from build123d import *

# Parameters (mm, degrees)
F1_DEPTH  = 9.652
F2_DEPTH  = 9.652
F4_DEPTH  = 44.704
F5_R      = 10.922
F7_DEPTH  = 3.175
F9_DEPTH  = 100.5007969078
F12_DEPTH = 3.175


with BuildPart() as f1:
    # F0 (on Top) → F1 (new body)
    with BuildSketch(Plane.XY):
        with BuildLine():
            Line((83.4274074162, 44.704), (19.9274074162, 44.704))
            Line((19.9274074162, 44.704), (19.9274074162, 0))
            Line((19.9274074162, 0), (83.4274074162, 0))
            Line((83.4274074162, 0), (83.4274074162, 12.7))
            Line((83.4274074162, 12.7), (58.0274074162, 12.7))
            ThreePointArc((58.0274074162, 12.7), (48.3754074162, 22.352), (58.0274074162, 32.004))
            Line((58.0274074162, 32.004), (83.4274074162, 32.004))
            Line((83.4274074162, 32.004), (83.4274074162, 44.704))
        make_face()
    extrude(amount=F1_DEPTH)

    # F0 (on Top) → F2 (join)
    with BuildSketch(Plane.XY):
        with BuildLine():
            ThreePointArc((83.4274074162, 0), (105.7794074162, 22.352), (83.4274074162, 44.704))
            Line((83.4274074162, 44.704), (83.4274074162, 32.004))
            ThreePointArc((83.4274074162, 32.004), (93.0794074162, 22.352), (83.4274074162, 12.7))
            Line((83.4274074162, 12.7), (83.4274074162, 0))
        make_face()
    extrude(amount=F2_DEPTH)

    # F3 (on face) → F4 (join)
    with BuildSketch(Plane.XZ):
        Polygon((19.9274074162, 0), (19.9274074162, 9.652), (0.8774074162, 42.6475678842), (-7.4814697811, 37.8215678842), (14.354822618, 0), align=None)
    extrude(amount=-F4_DEPTH)

    # F5
    f5_edges = [f1.edges().sort_by_distance(p)[0] for p in [
        (-3.302031, 0, 40.234568),
        (-3.302031, 44.704, 40.234568),
    ]]
    fillet(f5_edges, radius=F5_R)

    # F6 (on face) → F7 (cut)
    with BuildSketch(Plane(origin=(19.1249941608, 0, 11.041820527), x_dir=(0, 1, 0), z_dir=(0.8660254038, 0, 0.5))):
        with BuildLine():
            Line((17.272, 25.5731734892), (10.922, 25.5731734892))
            Line((10.922, 25.5731734892), (4.572, 25.5731734892))
            ThreePointArc((4.572, 25.5731734892), (10.922, 19.2231734892), (17.272, 25.5731734892))
        make_face()
        with BuildLine():
            Line((10.922, 31.9231734892), (10.922, 25.5731734892))
            Line((10.922, 25.5731734892), (17.272, 25.5731734892))
            ThreePointArc((17.272, 25.5731734892), (15.4121280605, 30.0633015498), (10.922, 31.9231734892))
        make_face()
        with BuildLine():
            Line((4.572, 25.5731734892), (10.922, 25.5731734892))
            Line((10.922, 25.5731734892), (10.922, 31.9231734892))
            ThreePointArc((10.922, 31.9231734892), (6.4318719395, 30.0633015498), (4.572, 25.5731734892))
        make_face()
        with BuildLine():
            ThreePointArc((33.782, 31.9231734892), (29.2918719395, 30.0633015498), (27.432, 25.5731734892))
            Line((27.432, 25.5731734892), (33.782, 25.5731734892))
            Line((33.782, 25.5731734892), (33.782, 31.9231734892))
        make_face()
        with BuildLine():
            Line((33.782, 31.9231734892), (33.782, 25.5731734892))
            Line((33.782, 25.5731734892), (40.132, 25.5731734892))
            ThreePointArc((40.132, 25.5731734892), (38.2721280605, 30.0633015498), (33.782, 31.9231734892))
        make_face()
        with BuildLine():
            Line((33.782, 25.5731734892), (27.432, 25.5731734892))
            ThreePointArc((27.432, 25.5731734892), (33.782, 19.2231734892), (40.132, 25.5731734892))
            Line((40.132, 25.5731734892), (33.782, 25.5731734892))
        make_face()
    extrude(amount=-F7_DEPTH, mode=Mode.SUBTRACT)

    # F8 (on face) → F9 (cut, through all)
    with BuildSketch(Plane(origin=(10.7661169635, 0, 6.215820527), x_dir=(0, -1, 0), z_dir=(-0.8660254038, 0, -0.5))):
        with BuildLine():
            Line((-30.607, 25.5731734892), (-33.782, 25.5731734892))
            Line((-33.782, 25.5731734892), (-36.957, 25.5731734892))
            ThreePointArc((-36.957, 25.5731734892), (-33.782, 22.3981734892), (-30.607, 25.5731734892))
        make_face()
        with BuildLine():
            Line((-33.782, 25.5731734892), (-33.782, 28.7481734892))
            ThreePointArc((-33.782, 28.7481734892), (-36.0270640303, 27.8182375195), (-36.957, 25.5731734892))
            Line((-36.957, 25.5731734892), (-33.782, 25.5731734892))
        make_face()
        with BuildLine():
            ThreePointArc((-30.607, 25.5731734892), (-31.5369359697, 27.8182375195), (-33.782, 28.7481734892))
            Line((-33.782, 28.7481734892), (-33.782, 25.5731734892))
            Line((-33.782, 25.5731734892), (-30.607, 25.5731734892))
        make_face()
        with BuildLine():
            Line((-10.922, 25.5731734892), (-10.922, 28.7481734892))
            ThreePointArc((-10.922, 28.7481734892), (-13.1670640303, 27.8182375195), (-14.097, 25.5731734892))
            Line((-14.097, 25.5731734892), (-10.922, 25.5731734892))
        make_face()
        with BuildLine():
            ThreePointArc((-7.747, 25.5731734892), (-8.6769359697, 27.8182375195), (-10.922, 28.7481734892))
            Line((-10.922, 28.7481734892), (-10.922, 25.5731734892))
            Line((-10.922, 25.5731734892), (-7.747, 25.5731734892))
        make_face()
        with BuildLine():
            Line((-10.922, 25.5731734892), (-14.097, 25.5731734892))
            ThreePointArc((-14.097, 25.5731734892), (-10.922, 22.3981734892), (-7.747, 25.5731734892))
            Line((-7.747, 25.5731734892), (-10.922, 25.5731734892))
        make_face()
    extrude(amount=-F9_DEPTH, mode=Mode.SUBTRACT)

    # F11 (on offset) → F12 (join, symmetric)
    with BuildSketch(Plane.XZ.offset(-22.352)):
        Polygon((0.8774074162, 42.6475678842), (19.9274074162, 9.652), (45.3274074162, 9.652), align=None)
    extrude(amount=F12_DEPTH, both=True)


solid = f1.part
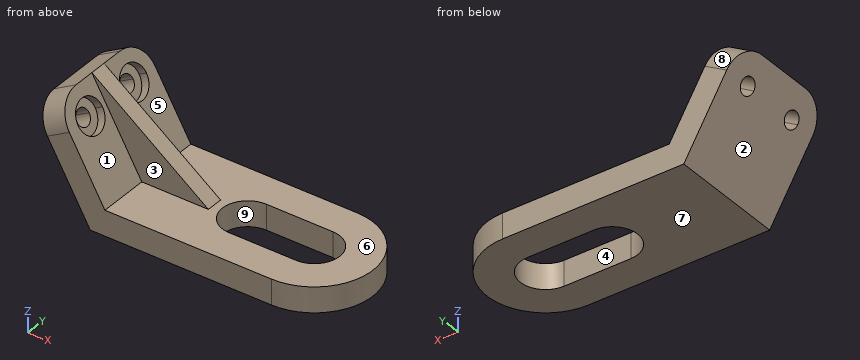
Here's how the part is built. I have some questions about the finished solid (model axes, mm). Face numbers are marked on the shaded views. A direction names the side the tool comes from. Give positions to 0.01 mm unless a question says otherwise; leave off trailing zeros. Loops run counter-clockwise (first coordinate to the right, second up) from the corner with the lowest first, then second, coordinate; pieces in that order, holes last. Notation, with made-up numbers: (11, 83.5) -> (37, 83.5) arc R20 cw to (37, 107.5) -> close; hole circle Ø9 at (-37.75, 73). An arc over 180 degrees is marked (long way). Answer as a JSON object with one key per item and string values. Group by question number.
Item 1: Thinking about a two-plate mould opening in X: for the marked faces 1, 2, 3 and 4, which applies, pulls with the +X half, pulls with the -X half, needs draft (parallel to the pull), parting line crosses it, or undercut?
Item 2: Imagine slicing it at A-A on x = 78.5. Write out the boundary of the cut face in (y, z), then the cut area to 3 significant figures.
Item 3: Imagine slicing it at B-B on y = 21. Write out the boundary of the cut face in (x, z), then the cut area to 3 significant figures.
Item 4: Imagine slicing it at D-D on x = 39.5. Write out the boundary of the cut face in (y, z).
Item 5: I need wall thicknesses on L1, parallel to Z at x = 31.5, y = 21.5; L2, parallel to Z at x = 21, y = 41; L3, parallel to Y at x = 74.5, z = 9. Which ranges of each line are inside material? Lowest first, please.
Item 6: On a 3-axis mill with a long thin cutter (end or side, diameter ignored), from which of +Z, -Z, +X, -X, +Y, -Y can I reach the whole of each face in a straight line? I mean the marked faces 5, 6, 7, 8 and 9. Say none if no direction works.
Item 7: Will these pins go through, and if not, where does the flat tip stop? pin 1 (10 mm diameter, centred on x = 30.5, z = 24.5, fed in from -Y); pin 2 (4 mm diameter, centred on y = 29, z = 26, fed in from +X); pin 3 (6 mm diameter, centred on y = 34.5, z = 31.5, fed in from -X).
Item 8: Imagine slicing it at C-C on z = 6.5. Write out the boundary of the cut face in (x, y).
Answer list:
{
 "1": {"face 1": "pulls with the +X half", "face 2": "pulls with the -X half", "face 3": "needs draft", "face 4": "undercut"},
 "2": {"outline": "(0, 0) -> (12.7, 0) -> (12.7, 9.65) -> (0, 9.65) -> close; (32, 0) -> (44.7, 0) -> (44.7, 9.65) -> (32, 9.65) -> close", "area": "245 mm2"},
 "3": {"outline": "(-7.48, 37.82) -> (14.35, 0) -> (48.47, 0) -> (48.47, 9.65) -> (45.33, 9.65) -> (0.88, 42.65) -> close; (92.98, 0) -> (105.74, 0) -> (105.74, 9.65) -> (92.98, 9.65) -> close", "area": "1,240 mm2"},
 "4": {"outline": "(0, 0) -> (44.7, 0) -> (44.7, 9.65) -> (25.53, 9.65) -> (25.53, 13.98) -> (19.18, 13.98) -> (19.18, 9.65) -> (0, 9.65) -> close"},
 "5": {"L1": "z = 0 to 19.92", "L2": "z = 0 to 9.65", "L3": "y = 0 to 12.7, 32 to 44.7"},
 "6": {"face 5": "+Z, +X, +Y", "face 6": "+Z, +X", "face 7": "-Z, +X, -X, +Y, -Y", "face 8": "+Z, -X, +Y", "face 9": "+Z, -Z"},
 "7": {"pin 1": "stops at y = 19.18", "pin 2": "stops at x = 11.64", "pin 3": "stops at x = -5.56"},
 "8": {"outline": "(10.6, 0) -> (83.43, 0) arc R22.35 ccw to (83.43, 44.7) -> (10.6, 44.7) -> close; hole (58.03, 12.7) -> (83.43, 12.7) arc R9.65 ccw to (83.43, 32) -> (58.03, 32) arc R9.65 ccw to start"}
}
